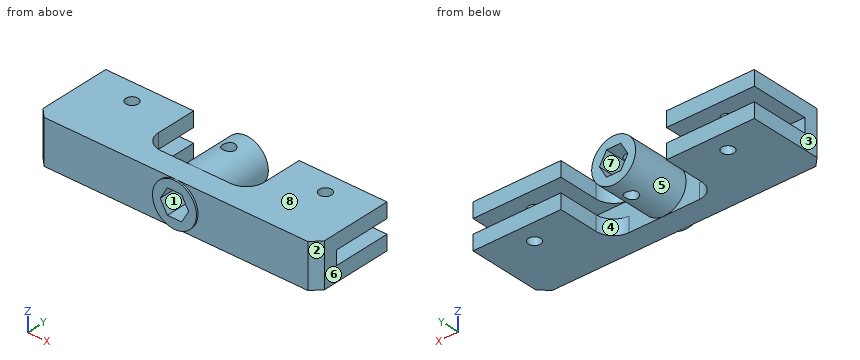
```python
from build123d import *
from build123d.topology import SkipClean

# Parameters (mm, degrees)
SKETCH1_R           = 6.25
BOSS_EXTRUDE1_DEPTH = 24
SKETCH2_R           = 1.75
CUT_EXTRUDE2_DEPTH  = 7.5
SKETCH3_W           = 80
SKETCH3_H           = 12.5
BOSS_EXTRUDE2_DEPTH = 7.5
CUT_EXTRUDE3_DEPTH  = 44.718560184
SKETCH5_W           = 80
SKETCH5_H           = 12.5
CUT_EXTRUDE4_DEPTH  = 1
BOSS_EXTRUDE3_START = -23.5
SKETCH6_R           = 6.25
BOSS_EXTRUDE3_DEPTH = 23.5
SKETCH7_W           = 25
SKETCH7_H           = 4.25
BOSS_EXTRUDE4_DEPTH = 16.5
FILLET1_R           = 5
SKETCH8_R           = 1.75
CUT_EXTRUDE5_DEPTH  = 7.5
LPATTERN1_COUNT     = 2
LPATTERN1_PITCH     = 27.5
LPATTERN1_COL_COUNT = 2
LPATTERN1_COL_PITCH = 27.5
CHAMFER1_SIZE       = 2.5


with BuildPart() as part:
    # Sketch1 → Boss-Extrude1 (new body)
    with BuildSketch(Plane(origin=(0, 0, 0), x_dir=(1, 0, 0), z_dir=(0, 1, 0))):
        with Locations(Location((0, 0, 0), (0, 0, 270))):
            Circle(SKETCH1_R)
        Polygon((4.041451884, 0), (2.020725942, 3.5), (-2.020725942, 3.5), (-4.041451884, 0), (-2.020725942, -3.5), (2.020725942, -3.5), align=None, mode=Mode.SUBTRACT)
    extrude(amount=BOSS_EXTRUDE1_DEPTH)

    # Sketch2 → Cut-Extrude2 (cut, symmetric)
    with BuildSketch(Plane.XY):
        with Locations((0, 17.746)):
            Circle(SKETCH2_R)
    extrude(amount=CUT_EXTRUDE2_DEPTH, both=True, mode=Mode.SUBTRACT)

    # Sketch3 → Boss-Extrude2 (add)
    with BuildSketch(Plane.XZ):
        Rectangle(SKETCH3_W, SKETCH3_H)
    extrude(amount=-BOSS_EXTRUDE2_DEPTH)

    # Sketch4 → Cut-Extrude3 (cut, through all)
    with BuildSketch(Plane(origin=(0, 7.5, 0), x_dir=(1, 0, 0), z_dir=(0, 1, 0))):
        Polygon((-2.020725942, -3.5), (2.020725942, -3.5), (4.041451884, 0), (2.020725942, 3.5), (-2.020725942, 3.5), (-4.041451884, 0), align=None)
    extrude(amount=-CUT_EXTRUDE3_DEPTH, mode=Mode.SUBTRACT)

    # Sketch5 → Cut-Extrude4 (cut)
    with BuildSketch(Plane.XZ):
        Rectangle(SKETCH5_W, SKETCH5_H)
    extrude(amount=-CUT_EXTRUDE4_DEPTH, mode=Mode.SUBTRACT)

    # Sketch6 → Boss-Extrude3 (add)
    with SkipClean():  # the faces are left unmerged after this step: merging them gives an invalid solid
        with BuildSketch(Plane(origin=(0, 24, 0), x_dir=(1, 0, 0), z_dir=(0, 1, 0)).offset(BOSS_EXTRUDE3_START)):
            with Locations(Location((0, 0, 0), (0, 0, 270))):
                Circle(SKETCH6_R)
            Polygon((-2.020725942, 3.5), (-4.041451884, 0), (-2.020725942, -3.5), (2.020725942, -3.5), (4.041451884, 0), (2.020725942, 3.5), align=None, mode=Mode.SUBTRACT)
        extrude(amount=BOSS_EXTRUDE3_DEPTH)
    add(part.part.scale(1), mode=Mode.REPLACE)  # the faces are merged on a copy

    # Sketch7 → Boss-Extrude4 (add)
    with BuildSketch(Plane(origin=(0, 7.5, 0), x_dir=(1, 0, 0), z_dir=(0, 1, 0))):
        with Locations((-27.5, 4.125)):
            Rectangle(SKETCH7_W, SKETCH7_H)
        with Locations((-27.5, -4.125)):
            Rectangle(SKETCH7_W, SKETCH7_H)
    boss_extrude4 = extrude(amount=BOSS_EXTRUDE4_DEPTH)

    # Mirror1: Boss-Extrude4 across plane
    add(boss_extrude4.mirror(Plane(origin=(0, 0, 0), x_dir=(0, 0, 1), z_dir=(1, 0, 0))))

    # Fillet1
    fillet1_edges = [part.edges().sort_by_distance(p)[0] for p in [
        (-15, 7.5, -4.125),
        (-15, 7.5, 4.125),
        (15, 7.5, -4.125),
        (15, 7.5, 4.125),
    ]]
    fillet(fillet1_edges, radius=FILLET1_R)

    # Sketch8 → Cut-Extrude5 (cut, symmetric)
    with BuildSketch(Plane.XY):
        with Locations((0, 18.246)):
            Circle(SKETCH8_R)
    cut_extrude5 = extrude(amount=CUT_EXTRUDE5_DEPTH, both=True, mode=Mode.SUBTRACT)

    # LPattern1: Cut-Extrude5 ×2
    with Locations(*[(i * LPATTERN1_PITCH, 0, 0) for i in range(1, LPATTERN1_COUNT)]):
        add(cut_extrude5, mode=Mode.SUBTRACT)

    # LPattern1 col: Cut-Extrude5 ×2
    with Locations(*[(-i * LPATTERN1_COL_PITCH, 0, 0) for i in range(1, LPATTERN1_COL_COUNT)]):
        add(cut_extrude5, mode=Mode.SUBTRACT)

    # Chamfer1
    chamfer1_edges = [part.edges().sort_by_distance(p)[0] for p in [
        (40, 1, 0),
        (-40, 1, 0),
    ]]
    chamfer(chamfer1_edges, length=CHAMFER1_SIZE)


solid = part.part
```
Here's how the part is built. I have some questions about the finished solid (model axes, mm). Face numbers are marked on the shaded views. A direction names the side the tool comes from. Round coordinates to 2 decimals unless told otherwise and drop trailing zeros. Order: outer loops, then holes, each group sorted by start corner. A loop starts at its lowest first (then second) coordinate and runs counter-clockwise, first axis right, second up. Notation, with made-up numbers: (24.5, -17) -> (62.5, -17) arc R23 ccw to (62.5, 18) -> close; hole circle Ø3 at (-25.5, -28.5). An arc over 180 degrees is marked (long way). Use a Markdown table: item, result. Add a question column.
(1) Suppose I cut it at B-B, the plane x = -27.5. Please give me the cut outline in (y, z).
(2) Suppose I cut it at C-C, the plane y = 13.5. Please give me the cut outline in (x, z), and give its area (3 significant figures).
(3) For pin 1 Ø4.5 at (x, y) = (0, 18.246) entering from -Z; pin 2 Ø1 at (x, y) = (-4, 14) entering from -Z; pin 3 Ø2 at (x, z) = (21.5, -2.5) entering from -Y; pin 4 Ø2 at (x, y) = (5.5, 19) entering from -Z, each with a flat end and sliding along its axis, tell me the tip position at first contact or that it passes through.
(4) If we mould it in two halves opening along Z, with no side actions, what happens to the marked faces 6, 7 and 8? For each: released by +Z, released by -Z, zero draft, split by the parting line, or undercut.
(5) Suppose I cut it at D-D, the plane z = -5.25. Please give me the cut outline in (x, y), and give its area (3 significant figures).
(6) I need wall thicknesses on line 1 along Y through (x, z) = (27.5, 5.15); line 2 along Z through (x, y) = (27.5, 12.75); line 3 along X through (y, z) = (20.75, 5). Which ranges of each line are inside material? Lowest first, please.
(7) Suppose I cut it at A-A, the plane y = 8.5. Please give me the cut outline in (x, z), and give its area (3 significant figures).
(8) For the marked faces 1, 2, 3, 4 and 5, which set-ups out of +Z, -Z, +X, -X, +Y, -Y let a thin tool reach every point of the face, with its end or its side?
Verdict:
| question | item | result |
|---|---|---|
| 1 | outline | (1, -6.25) -> (16.5, -6.25) -> (16.5, -2) -> (7.5, -2) -> (7.5, 2) -> (16.5, 2) -> (16.5, 6.25) -> (1, 6.25) -> close; (20, -6.25) -> (24, -6.25) -> (24, -2) -> (20, -2) -> close; (20, 2) -> (24, 2) -> (24, 6.25) -> (20, 6.25) -> close |
| 2 | outline | (-40, -6.25) -> (-15, -6.25) -> (-15, -2) -> (-40, -2) -> close; (-40, 2) -> (-15, 2) -> (-15, 6.25) -> (-40, 6.25) -> close; circle Ø12.5 at (0, 0); (15, -6.25) -> (40, -6.25) -> (40, -2) -> (15, -2) -> close; (15, 2) -> (40, 2) -> (40, 6.25) -> (15, 6.25) -> close; hole (-4.04, 0) -> (-2.02, -3.5) -> (2.02, -3.5) -> (4.04, 0) -> (2.02, 3.5) -> (-2.02, 3.5) -> close |
| 2 | area | 505 mm2 |
| 3 | pin 1 | z = -6.25 |
| 3 | pin 2 | z = -5.18 |
| 3 | pin 3 | y = 1 |
| 3 | pin 4 | z = -4.34 |
| 4 | face 6 | zero draft |
| 4 | face 7 | undercut |
| 4 | face 8 | released by +Z |
| 5 | outline | (-40, 3.5) -> (-37.5, 1) -> (-3.39, 1) -> (-3.39, 0.5) -> (3.39, 0.5) -> (3.39, 1) -> (37.5, 1) -> (40, 3.5) -> (40, 24) -> (15, 24) -> (15, 12.5) arc R5 cw to (10, 7.5) -> (3.39, 7.5) -> (3.39, 24) -> (-3.39, 24) -> (-3.39, 7.5) -> (-10, 7.5) arc R5 cw to (-15, 12.5) -> (-15, 24) -> (-40, 24) -> close; hole circle Ø3.5 at (-27.5, 18.25); hole circle Ø3.5 at (0, 18.25); hole circle Ø3.5 at (27.5, 18.25) |
| 5 | area | 1,440 mm2 |
| 6 | line 1 | 1 to 16.5, 20 to 24 |
| 6 | line 2 | -6.25 to -2, 2 to 6.25 |
| 6 | line 3 | -40 to -15, -3.75 to 3.75, 15 to 40 |
| 7 | outline | (-40, -6.25) -> (-13, -6.25) -> (-13, -2) -> (-40, -2) -> close; (-40, 2) -> (-13, 2) -> (-13, 6.25) -> (-40, 6.25) -> close; circle Ø12.5 at (0, 0); (13, -6.25) -> (40, -6.25) -> (40, -2) -> (13, -2) -> close; (13, 2) -> (40, 2) -> (40, 6.25) -> (13, 6.25) -> close; hole (-4.04, 0) -> (-2.02, -3.5) -> (2.02, -3.5) -> (4.04, 0) -> (2.02, 3.5) -> (-2.02, 3.5) -> close |
| 7 | area | 539 mm2 |
| 8 | face 1 | +Y, -Y |
| 8 | face 2 | +Z, -Z, +X, -Y |
| 8 | face 3 | +Z, -Z, -X, +Y, -Y |
| 8 | face 4 | +Z, -Z, +Y |
| 8 | face 5 | +Y |
